from build123d import *

# Parameters (mm, degrees)
SKETCH2_W           = 3.5
SKETCH2_H           = 4.5
BOSS_EXTRUDE1_DEPTH = 7
SKETCH3_R           = 3.5
BOSS_EXTRUDE2_DEPTH = 7
CUT_EXTRUDE1_DEPTH  = 5
FILLET1_R           = 0.2
FILLET2_R           = 0.2


with BuildPart() as part:
    # Sketch2 → Boss-Extrude1 (new body)
    with BuildSketch(Plane(origin=(0, 0, 0), x_dir=(0, 1, 0), z_dir=(0, 0, 1))):
        with Locations((1.75, 2.25)):
            Rectangle(SKETCH2_W, SKETCH2_H)
    extrude(amount=BOSS_EXTRUDE1_DEPTH)

    # Sketch3 → Boss-Extrude2 (add)
    with BuildSketch(Plane.XY.offset(7)):
        with Locations((-2.25, 1.75)):
            Circle(SKETCH3_R)
    extrude(amount=BOSS_EXTRUDE2_DEPTH)

    # Sketch4 → Cut-Extrude1 (cut)
    with BuildSketch(Plane.XY.offset(14)):
        Polygon((-3.35, 2.85), (-4.85, 2.85), (-4.85, 0.65), (-3.35, 0.65), (-3.35, -0.85), (-1.15, -0.85), (-1.15, 0.65), (0.35, 0.65), (0.35, 3.05), (-1.15, 3.05), (-1.15, 4.35), (-3.35, 4.35), align=None)
    extrude(amount=-CUT_EXTRUDE1_DEPTH, mode=Mode.SUBTRACT)

    # Fillet1
    fillet1_edges = [part.edges().sort_by_distance(p)[0] for p in [
        (0, 3.5, 3.5),
    ]]
    fillet(fillet1_edges, radius=FILLET1_R)

    # Fillet2
    fillet2_edges = [part.edges().sort_by_distance(p)[0] for p in [
        (-4.5, 0, 3.5),
        (-4.5, 3.5, 3.5),
        (0, 0, 3.5),
    ]]
    fillet(fillet2_edges, radius=FILLET2_R)


solid = part.part
Build history of the part. All positions in model axes, mm. A direction names the side the tool comes from. Coordinates: 2 decimals unless noted, no trailing zeros. Order: outer loops, then holes, each group sorted by start corner. A loop starts at its lowest first (then second) coordinate and runs counter-clockwise, first axis right, second up. Notation, with made-up numbers: (-39, -7.5) - (17, -7.5) arc R18 cw to (17, -2.5) - close; hole circle Ø7 at (72.5, -6). An arc over 180 degrees is marked (long way). Write each question's results on one line, items separated by ' | '. Start each with the question number.
Item 1: Wall check: probe 1 along Y at (x, z) = (-4.25, 1); probe 2 along X at (y, z) = (2.25, 4); probe 3 along Z at (x, y) = (-2.5, -0.5). Give the ranges that are in metal, low to high. Write a range as [from, to].
Item 2: Band-saw the part on A-A on y = 1.75. Write the cut outline in (x, z).
Item 3: Band-saw the part on C-C on x = -2.25. Write the cut outline in (y, z), and give its area (3 significant figures).
Item 4: Band-saw the part on B-B on z = 12.75. Write the cut outline in (x, y).
Item 5: Band-saw the part on D-D on z = 6.25. Write the cut outline in (x, y).
Item 6: Mould opens along Y. For faces 5 (the face through (0, 0.65, 12)), 6 (the face through (-2, 0, 3)), 7 (the face through (-4.5, 2, 3)) say: released by +Y, released by -Y, zero draft, split by the parting line, or undercut.
Item 7: Flat gauge pins, fed straight in: pin 1 (1 mm diameter, centred on y = 0.5, z = 9, fed in from -X); pin 2 (1.2 mm diameter, centred on y = -0.5, z = 11, fed in from -X); pin 3 (1.6 mm diameter, centred on y = -0.5, z = 10.5, fed in from +X). Where does each tip first touch, or does it go through?
Item 8: Tool access for faces 1 (the face through (-3.35, 0, 12)), 2 (the face through (-2, 3.5, 3)), 3 (the face through (0, 2, 3)), 4 (the face through (-2, -1, 7)): list every direction of +Z, -Z, +X, -X, +Y, -Y with a clear straight run to the whole face (end or side of a thin tool).
Numbers:
1) probe 1: [0, 3.5] | probe 2: [-4.5, 0] | probe 3: [7, 9]
2) outline: (-5.75, 7) - (-4.5, 7) - (-4.5, 0) - (0, 0) - (0, 7) - (1.25, 7) - (1.25, 14) - (0.35, 14) - (0.35, 9) - (-4.85, 9) - (-4.85, 14) - (-5.75, 14) - close
3) outline: (-1.75, 7) - (0, 7) - (0, 0) - (3.5, 0) - (3.5, 7) - (5.25, 7) - (5.25, 14) - (4.35, 14) - (4.35, 9) - (-0.85, 9) - (-0.85, 14) - (-1.75, 14) - close | area: 47.5 mm^2
4) outline: circle Ø7 at (-2.25, 1.75); hole (-4.85, 0.65) - (-3.35, 0.65) - (-3.35, -0.85) - (-1.15, -0.85) - (-1.15, 0.65) - (0.35, 0.65) - (0.35, 3.05) - (-1.15, 3.05) - (-1.15, 4.35) - (-3.35, 4.35) - (-3.35, 2.85) - (-4.85, 2.85) - close
5) outline: (-4.5, 0.2) arc R0.2 ccw to (-4.3, 0) - (-0.2, 0) arc R0.2 ccw to (0, 0.2) - (0, 3.3) arc R0.2 ccw to (-0.2, 3.5) - (-4.3, 3.5) arc R0.2 ccw to (-4.5, 3.3) - close
6) face 5: undercut | face 6: released by -Y | face 7: zero draft
7) pin 1: x = -5.67 | pin 2: x = -5.34 | pin 3: x = 0.94
8) face 1: +Z | face 2: -Z, +X, -X, +Y | face 3: -Z, +X, +Y, -Y | face 4: -Z
